CAD build for the part. Positions are in the model's coordinates, mm. Face numbers are marked on the shaded views. Round coordinates to 2 decimals unless told otherwise and drop trailing zeros. Loops run counter-clockwise (first coordinate to the right, second up) from the corner with the lowest first, then second, coordinate; pieces in that order, holes last. Notation, with made-up numbers: M 31.5,-34 L 43.5,-34 A8 ccw 43.5,-20 Z; hole C 62.5,19 d11. An arc over 180 degrees is marked long. Use one line per item in the form item = value.
from build123d import *

# Parameters (mm, degrees)
CROQUIS1_R              = 2.6
CROQUIS1_R_2            = 1.7
SALIENTE_EXTRUIR1_DEPTH = 7


with BuildPart() as part:
    # Croquis1 → Saliente-Extruir1 (new body)
    with BuildSketch(Plane.XY):
        with BuildLine():
            Line((2.811164445, 2.891458498), (9.18120322, -3.301688153))
            ThreePointArc((9.18120322, -3.301688153), (9.762664554, -4.15232303), (9.967236954, -5.162187927))
            Line((9.967236954, -5.162187927), (9.967236954, -10))
            Line((9.967236954, -10), (-4.032763046, -10))
            Line((-4.032763046, -10), (-4.032763046, 0))
            ThreePointArc((-4.032763046, 0), (-1.569461324, 3.714830944), (2.811164445, 2.891458498))
        make_face()
        Circle(CROQUIS1_R, mode=Mode.SUBTRACT)
        with Locations((7.372368399, -5.162187927)):
            Circle(CROQUIS1_R_2, mode=Mode.SUBTRACT)
    extrude(amount=SALIENTE_EXTRUIR1_DEPTH)


solid = part.part
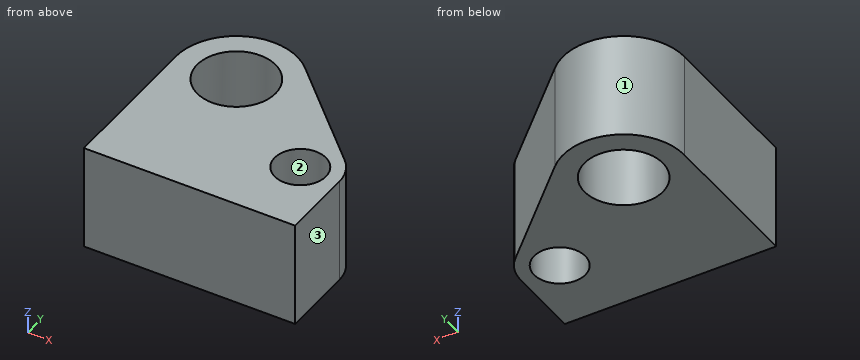
1. Cut at A-A on x = 0. Write the cut outline in (y, z).
Completed:
outline = M -10,0 L -2.6,0 L -2.6,7 L -10,7 Z; M 2.6,0 L 4.03,0 L 4.03,7 L 2.6,7 Z
2. Pull direction X, two halves, no side cores. Call the marked faces 1, 2 and 3: +X half, -X half, draft (parallel to the pull), parting line (faces both ways), or undercut.
Completed:
face_1 = parting line
face_2 = undercut
face_3 = +X half
3. Probe line 1 along Y through (x, z) = (0, 2); line 2 along X through (y, z) = (-1, 4); line 3 along X through (y, z) = (-5, 3.5). List the from-to ranges inside material, lowest first. Write a range as from..to.
Completed:
line_1 = -10..-2.6, 2.6..4.03
line_2 = -4.03..-2.4, 2.4..6.81
line_3 = -4.03..5.68, 9.06..9.96
4. Cut at C-C on y = -4.75. Write the cut outline in (x, z), and give its area (3 significant figures).
Completed:
outline = M -4.03,0 L 5.72,0 L 5.72,7 L -4.03,7 Z; M 9.02,0 L 9.93,0 L 9.93,7 L 9.02,7 Z
area = 74.7 mm2
5. Cut at D-D on x = 3.5. Write the cut outline in (y, z), and give its area (3 significant figures).
Completed:
outline = M -10,0 L 2.22,0 L 2.22,7 L -10,7 Z
area = 85.6 mm2
6. Cut at B-B on z = 3. Write the cut outline in (x, y).
Completed:
outline = M -4.03,-10 L 9.97,-10 L 9.97,-5.16 A2.59 ccw 9.18,-3.3 L 2.81,2.89 A4.03 ccw -4.03,0 Z; hole C 0,0 d5.2; hole C 7.37,-5.16 d3.4
